For this review, take the finished solid that the model builds, in its own axes (mm). A direction names the side the tool comes from. Round coordinates to 2 decimals unless told otherwise and drop trailing zeros. Write each loop counter-clockwise with the first axis right and the second up, starting at its lowest first coordinate (ties: lowest second). Pieces come first, ordered by that corner, then holes.
from build123d import *

# Parameters (mm, degrees)
F1_DEPTH = 25.4
F2_DEPTH = 762
F3_R     = 304.8
F4_DEPTH = 431.8


with BuildPart() as f1:
    # F0 (on Front) → F1 (new body)
    with BuildSketch(Plane.XZ):
        Polygon((571.5, -88.9), (304.8, 190.5), (-304.8, 190.5), (-571.5, -88.9), (-571.5, -190.5), (571.5, -190.5), align=None)
    extrude(amount=F1_DEPTH)

    # F0 (on Front) → F2 (join)
    with BuildSketch(Plane.XZ):
        Polygon((571.5, -88.9), (304.8, 190.5), (-304.8, 190.5), (-571.5, -88.9), (-571.5, -190.5), (571.5, -190.5), align=None)
    extrude(amount=F2_DEPTH)

    # F3 (on face) → F4 (join)
    with BuildSketch(Plane.XY.offset(190.5)):
        with Locations((0, -381)):
            Circle(F3_R)
        with BuildLine():
            ThreePointArc((-304.8, -381), (0, -685.8), (304.8, -381))
            ThreePointArc((304.8, -381), (0, -76.2), (-304.8, -381))
        make_face()
    extrude(amount=F4_DEPTH)


solid = f1.part
(1) We need section C-C, the plane z = 444. Give the boundary of the cut face in (x, y), and give its area (3 significant figures).
Geometry check:
outline: circle Ø609.6 at (0, -381)
area: 292,000 mm2
(2) For pin 1 Ø5 at (y, z) = (-107.5, 142.5) entering from -X, flat-tipped, find the tip position at first contact; note if it passes through.
Geometry check:
pin 1: stops at x = -353
(3) We need section A-A, the plane x = 0. Give the boundary of the cut face in (y, z).
Geometry check:
outline: (-762, -190.5) - (0, -190.5) - (0, 190.5) - (-76.2, 190.5) - (-76.2, 622.3) - (-685.8, 622.3) - (-685.8, 190.5) - (-762, 190.5) - close
(4) We need section B-B, the plane y = -185. Give the boundary of the cut face in (x, z).
Geometry check:
outline: (-571.5, -190.5) - (571.5, -190.5) - (571.5, -88.9) - (304.8, 190.5) - (233.42, 190.5) - (233.42, 622.3) - (-233.42, 622.3) - (-233.42, 190.5) - (-304.8, 190.5) - (-571.5, -88.9) - close
(5) We need section D-D, the plane x = 198.5. Give the boundary of the cut face in (y, z), and give its area (3 significant figures).
Geometry check:
outline: (-762, -190.5) - (0, -190.5) - (0, 190.5) - (-149.7, 190.5) - (-149.7, 622.3) - (-612.3, 622.3) - (-612.3, 190.5) - (-762, 190.5) - close
area: 490,000 mm2
(6) For faces 1 (the face through (-8, -376, -190.5)), 2 (the face through (-66.075, -678.552, 403.377)), 3 (the face through (-571.5, -376, -139)), 4 (the face through (4, -61, 190.5)), 5 (the face through (1, -698, 190.5)), list the 3-axis set-ups (+Z, -Z, +X, -X, +Y, -Y) from which the entire face can be reached by the end or side of a thin tool; tool diameter is ignored.
Geometry check:
face 1: -Z, +X, -X, +Y, -Y
face 2: +Z
face 3: +Z, -Z, -X, +Y, -Y
face 4: +Z, +Y
face 5: +Z, -Y
(7) For line 1 along Z through (x, y) = (108, -717); line 2 along Z through (x, y) = (-450, -383); line 3 along X through (y, z) = (-536, 451.5), list the stretches that pass through material, from the lowest coordinate up.
Geometry check:
line 1: z = -190.5 to 190.5
line 2: z = -190.5 to 38.39
line 3: x = -262.45 to 262.45
